The model under review builds one solid part; all positions refer to its coordinate system, in mm. Face numbers are marked on the shaded views. A direction names the side the tool comes from. Give positions to 0.01 mm unless a question says otherwise; leave off trailing zeros. Loops run counter-clockwise (first coordinate to the right, second up) from the corner with the lowest first, then second, coordinate; pieces in that order, holes last. Notation, with made-up numbers: (-31, -31) - (-25, -31) arc R16 ccw to (-25, -19) - close; hole circle Ø4 at (45.5, -20.75). An arc over 180 degrees is marked (long way). Answer as a JSON object with one key per item and string values.
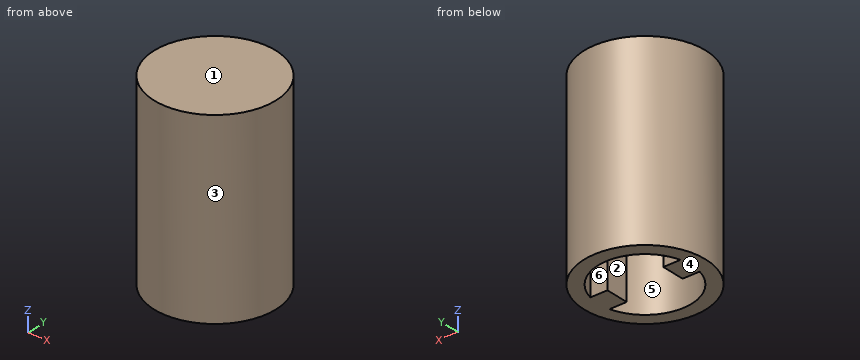
from build123d import *

# Parameters (mm, degrees)
F1_R     = 6.5
F2_DEPTH = 20
F3_DEPTH = 15


with BuildPart() as f2:
    # F1 (on Top) → F2 (new body)
    with BuildSketch(Plane.XY):
        Circle(F1_R)
    extrude(amount=F2_DEPTH)

    # F0 (on Top) → F3 (cut)
    with BuildSketch(Plane.XY):
        with BuildLine():
            Line((3, 0), (3, 1.25))
            Line((3, 1.25), (4.841229, 1.25))
            ThreePointArc((4.841229, 1.25), (0, 5), (-4.841229, 1.25))
            Line((-4.841229, 1.25), (-3, 1.25))
            Line((-3, 1.25), (-3, 0))
            Line((-3, 0), (-3, -1.25))
            Line((-3, -1.25), (-4.841229, -1.25))
            ThreePointArc((-4.841229, -1.25), (0, -5), (4.841229, -1.25))
            Line((4.841229, -1.25), (3, -1.25))
            Line((3, -1.25), (3, 0))
        make_face()
    extrude(amount=F3_DEPTH, mode=Mode.SUBTRACT)


solid = f2.part
Q1. For the marked faces 1 and 2, list the 3-axis set-ups (+Z, -Z, +X, -X, +Y, -Y) from which the entire face can be reached by the end or side of a thin tool; tool diameter is ignored.
Results:
{"face 1": "+Z, +X, -X, +Y, -Y", "face 2": "-Z"}
Q2. The part is to be moulded in two halves that separate along Y. For the marked faces 3, 4, 5 and 6, say which applies: +Y half, -Y half, draft (parallel to the pull), parting line (faces both ways), or undercut.
Results:
{"face 3": "parting line", "face 4": "draft", "face 5": "undercut", "face 6": "undercut"}
Q3. Consider section B-B, the plane x = 0. State the section outline as (y, z) points.
Results:
{"outline": "(-6.5, 0) - (-5, 0) - (-5, 15) - (5, 15) - (5, 0) - (6.5, 0) - (6.5, 20) - (-6.5, 20) - close"}
Q4. Consider section C-C, the plane y = -3. State the section outline as (x, z) points, plus the area to 3 significant figures.
Results:
{"outline": "(-5.77, 0) - (-4, 0) - (-4, 15) - (4, 15) - (4, 0) - (5.77, 0) - (5.77, 20) - (-5.77, 20) - close", "area": "111 mm^2"}
Q5. Consider section D-D, the plane z = 18.75. State the section outline as (x, y) points, plus the area to 3 significant figures.
Results:
{"outline": "circle Ø13 at (0, 0)", "area": "133 mm^2"}
Q6. Consider section A-A, the plane z = 8. State the section outline as (x, y) points.
Results:
{"outline": "circle Ø13 at (0, 0); hole (-4.84, -1.25) arc R5 ccw to (4.84, -1.25) - (3, -1.25) - (3, 1.25) - (4.84, 1.25) arc R5 ccw to (-4.84, 1.25) - (-3, 1.25) - (-3, -1.25) - close"}
Q7. Clearance check with flat-ended pins moving along their axes: pin 1 Ø0.6 at (x, z) = (-4, 7) entering from -Y; pin 2 Ø2 at (x, z) = (-4, 9.5) entering from +Y; pin 3 Ø3 at (x, y) = (0.5, 1.5) entering from -Z. State where each tip first meets the part, or that it passes through.
Results:
{"pin 1": "stops at y = -5.34", "pin 2": "stops at y = 5.77", "pin 3": "stops at z = 15"}
Q8. To check wall thickness, follow probe 1 along X at (y, z) = (0.25, 12); probe 2 along Y at (x, z) = (-3.75, 4.5); probe 3 along X at (y, z) = (2, 3.5). State the ranges of each line that lie inside material, in increasing order. Write a range as [from, to].
Results:
{"probe 1": "x = [-6.5, -3], [3, 6.5]", "probe 2": "y = [-5.31, -3.31], [-1.25, 1.25], [3.31, 5.31]", "probe 3": "x = [-6.18, -4.58], [4.58, 6.18]"}
